```python
from build123d import *

# Parameters (mm, degrees)
BOSS_EXTRUDE1_DEPTH = 25
SKETCH5_W           = 8.5
SKETCH5_H           = 8.5
CUT_EXTRUDE1_DEPTH  = 20
SKETCH6_R           = 1.75
CUT_EXTRUDE2_DEPTH  = 13
SKETCH7_R           = 1.75
CUT_EXTRUDE3_DEPTH  = 13
SKETCH8_W           = 32
SKETCH8_H           = 19.425554826
SKETCH8_R           = 1.75
BOSS_EXTRUDE2_DEPTH = 3
CHAMFER3_SIZE       = 5


with BuildPart() as part:
    # Sketch2 → Boss-Extrude1 (new body)
    with BuildSketch(Plane(origin=(0, 0, 0), x_dir=(1, 0, 0), z_dir=(0, 1, 0))):
        Polygon((0, 0), (0, 13.5), (2.962777413, 16.462777413), (21.462777413, 16.462777413), (24.425554826, 13.5), (24.425554826, 0), (21.462777413, -2.962777413), (2.962777413, -2.962777413), align=None)
    extrude(amount=BOSS_EXTRUDE1_DEPTH)

    # Sketch5 → Cut-Extrude1 (cut)
    with BuildSketch(Plane(origin=(0, 0, 0), x_dir=(-1, 0, 0), z_dir=(0, -1, 0))):
        with Locations((-7.962777413, 11.212777413)):
            Rectangle(SKETCH5_W, SKETCH5_H)
        with Locations((-16.462777413, 2.287222587)):
            Rectangle(SKETCH5_W, SKETCH5_H)
    extrude(amount=-CUT_EXTRUDE1_DEPTH, mode=Mode.SUBTRACT)

    # Sketch6 → Cut-Extrude2 (cut)
    with BuildSketch(Plane(origin=(0, 20, 0), x_dir=(-1, 0, 0), z_dir=(0, -1, 0))):
        with Locations(Location((-7.962777413, 11.212777413, 0), (0, 0, 90))):
            Circle(SKETCH6_R)
    extrude(amount=-CUT_EXTRUDE2_DEPTH, mode=Mode.SUBTRACT)

    # Sketch7 → Cut-Extrude3 (cut)
    with BuildSketch(Plane.XZ.offset(-20)):
        with Locations(Location((16.462777413, -2.287222587, 0), (0, 0, 270))):
            Circle(SKETCH7_R)
    extrude(amount=-CUT_EXTRUDE3_DEPTH, mode=Mode.SUBTRACT)

    # Sketch8 → Boss-Extrude2 (add)
    with BuildSketch(Plane(origin=(0, 25, 0), x_dir=(1, 0, 0), z_dir=(0, 1, 0))):
        with Locations((12.212777413, 6.75)):
            Rectangle(SKETCH8_W, SKETCH8_H)
        with Locations(Location((7.962777413, 11.212777413, 0), (0, 0, 90))):
            Circle(SKETCH8_R, mode=Mode.SUBTRACT)
        with Locations(Location((16.462777413, 2.287222587, 0), (0, 0, 90))):
            Circle(SKETCH8_R, mode=Mode.SUBTRACT)
    extrude(amount=BOSS_EXTRUDE2_DEPTH)

    # Chamfer3
    chamfer3_edges = [part.edges().sort_by_distance(p)[0] for p in [
        (28.212777413, 26.5, 2.962777413),
        (28.212777413, 26.5, -16.462777413),
        (-3.787222587, 26.5, -16.462777413),
        (-3.787222587, 26.5, 2.962777413),
    ]]
    chamfer(chamfer3_edges, length=CHAMFER3_SIZE)


solid = part.part
```
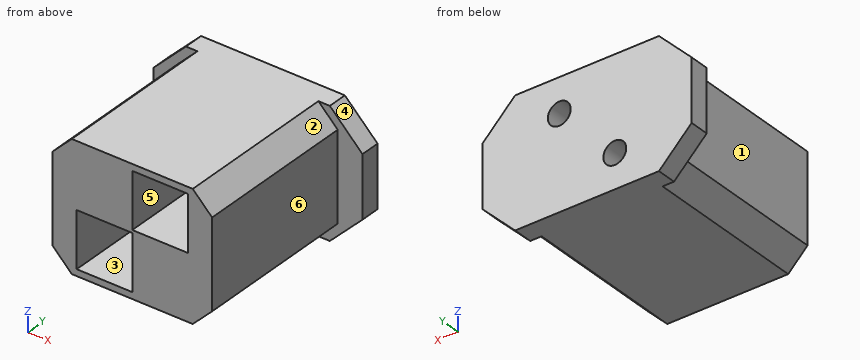
The listing builds one solid part. Answer for the finished solid, in the listing's coordinates (mm). Face numbers are marked on the shaded views. A direction names the side the tool comes from. Coordinates: 2 decimals unless noted, no trailing zeros. Write each loop counter-clockwise with the first axis right and the second up, starting at its lowest first coordinate (ties: lowest second). Pieces come first, ordered by that corner, then holes.
Q1. Section C-C, the plane x = 16 is taken. Write down the section's boundary in (y, z), then the cut area to 3 significant figures.
Returned:
outline: (0, -16.46) - (28, -16.46) - (28, -3.97) - (20, -3.97) - (20, -6.54) - (0, -6.54) - close; (0, 1.96) - (20, 1.96) - (20, -0.6) - (28, -0.6) - (28, 2.96) - (0, 2.96) - close
area: 347 mm2
Q2. Find the intervals of material crossed by line 1 along X through (y, z) = (3.5, -13); line 2 along Z through (x, y) = (19, 11.75); line 3 along X through (y, z) = (10.5, -1), in increasing order.
Returned:
line 1: x = 0 to 3.71, 12.21 to 24.43
line 2: z = -16.46 to -6.54, 1.96 to 2.96
line 3: x = 0 to 12.21, 20.71 to 24.43
Q3. Section B-B, the plane z = -8.75 is taken. Write down the section's boundary in (x, y).
Returned:
outline: (-3.79, 25) - (0, 25) - (0, 0) - (3.71, 0) - (3.71, 20) - (12.21, 20) - (12.21, 0) - (24.43, 0) - (24.43, 25) - (28.21, 25) - (28.21, 28) - (-3.79, 28) - close
Q4. Section D-D, the plane z = -12.25 is taken. Write down the section's boundary in (x, y), then the cut area to 3 significant figures.
Returned:
outline: (-3, 25) - (0, 25) - (0, 0) - (3.71, 0) - (3.71, 20) - (6.55, 20) - (6.55, 28) - (-3, 28) - close; (9.37, 20) - (12.21, 20) - (12.21, 0) - (24.43, 0) - (24.43, 25) - (27.43, 25) - (27.43, 28) - (9.37, 28) - close
area: 509 mm2
Q5. The mould has two halves that part along Z. Classify the marked faces 4, 5 and 6: released by +Z, released by -Z, zero draft, split by the parting line, or undercut.
Returned:
face 4: released by +Z
face 5: undercut
face 6: zero draft
Q6. Given P1, Ø4, axis at y = 12, z = -13.5, coming from the -X side; P2, Ø2.5, axis at x = 15.5, z = -2.5, coming from the -Y side; P3, Ø7, axis at y = 7, z = -4, coming from the +X side, each flat-ended and moving along its own axis, determine where each tip first touches the part or whether it passes through.
Returned:
P1: stops at x = 0
P2: stops at y = 20
P3: stops at x = 24.43
Q7. Section A-A, the plane y = 7.75 is taken. Write down the section's boundary in (x, z).
Returned:
outline: (0, -13.5) - (2.96, -16.46) - (21.46, -16.46) - (24.43, -13.5) - (24.43, 0) - (21.46, 2.96) - (2.96, 2.96) - (0, 0) - close; hole (3.71, -15.46) - (12.21, -15.46) - (12.21, -6.96) - (3.71, -6.96) - close; hole (12.21, -6.54) - (20.71, -6.54) - (20.71, 1.96) - (12.21, 1.96) - close
Q8. Which of the six approach directions +Z, -Z, +X, -X, +Y, -Y give full straight-line access (tool end or side, diameter ignored) to the marked faces 1, 2 and 3?
Returned:
face 1: +Z, -Z, -X, -Y
face 2: +Z, +X, -Y
face 3: -Y
